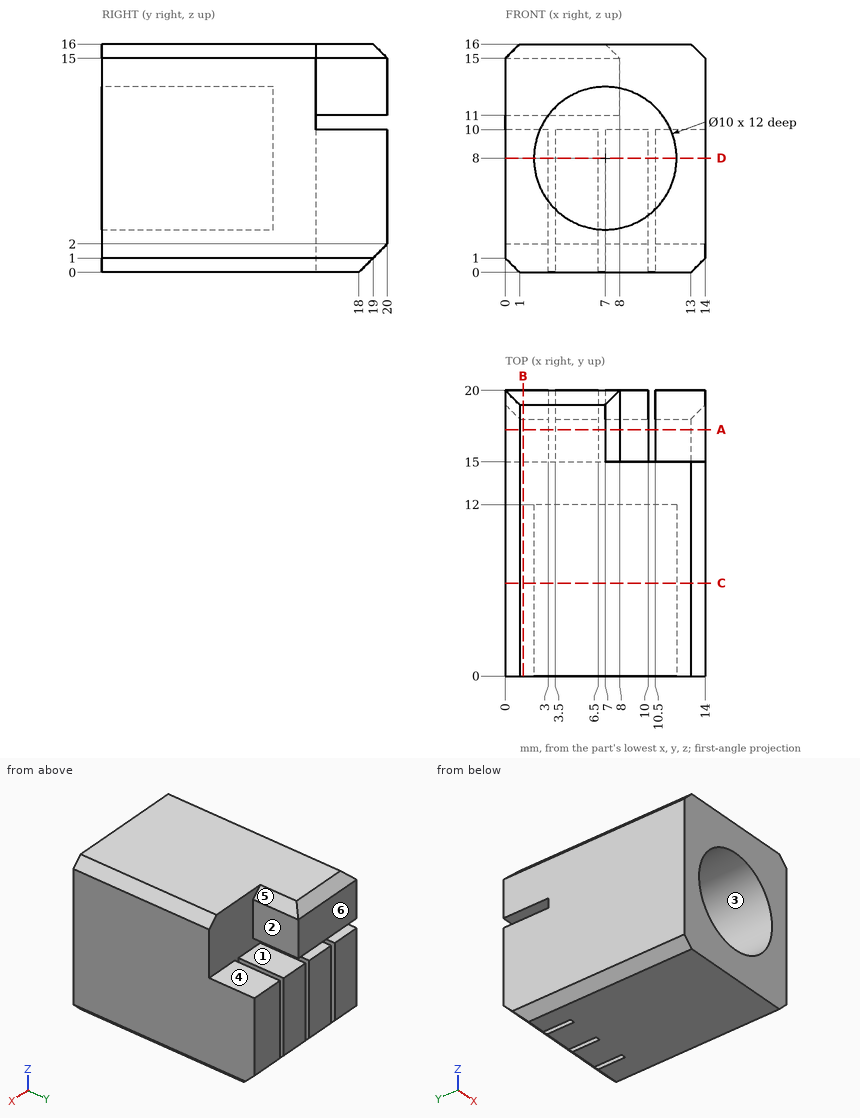
Job drawing, mm, ordinate dimensions from the low corner. One solid piece. A direction names the side the tool comes from. Round coordinates to 2 decimals unless told otherwise and drop trailing zeros. Loops run counter-clockwise (first coordinate to the right, second up) from the corner with the lowest first, then second, coordinate; pieces in that order, holes last. Notation, with made-up numbers: M -11.75,85.5 L 13.25,85.5 A14 cw 13.25,96.5 Z; hole C 15,-12.75 d2. An arc over 180 degrees is marked long. One line per question, with ' | ' between items. Start each with the question number.
Item 1: Two-plate mould, pull along X, no slides. Class the marked faces 1, 2 and 3: pulls with the +X half, pulls with the -X half, needs draft (parallel to the pull), parting line crosses it, or undercut.
Item 2: Pin check, flat tips, straight feed: pin 1 Ø1.8 at (x, y) = (12.5, 16.5) entering from +Z; pin 2 Ø5 at (x, y) = (4.5, 9.5) entering from -Z; pin 3 Ø1.5 at (x, z) = (11.5, 12) entering from +Y; pin 4 Ø3 at (y, z) = (18, 13.5) entering from +X. Stop position of each tip, or through.
Item 3: Which spindle directions (+Z, -Z, +X, -X, +Y, -Y) get a long thin tool onto all of the face, cutting with end or side? Do the marked faces 4, 5 and 6. Say none if no direction does.
Item 4: Cut at B-B, the plane x = 1.25. Write the cut outline in (y, z).
Item 5: Cut at A-A, the plane y = 17.25. Write the cut outline in (x, z), plus the area to 3 significant figures.
Item 6: Wall check: line 1 (X direction, y = 5.5, z = 8.25); line 2 (Z direction, x = 3, y = 2.5); line 3 (X direction, y = 3.5, z = 10.75). Give the ranges that are in metal, low to high.
Item 7: Cut at C-C, the plane y = 6.5. Write the cut outline in (x, z).
Item 8: Cut at D-D, the plane z = 8. Write the cut outline in (x, y).
Responses:
1) face 1: needs draft | face 2: pulls with the +X half | face 3: undercut
2) pin 1: stops at z = 10 | pin 2: stops at z = 0 | pin 3: stops at y = 15 | pin 4: stops at x = 8
3) face 4: +Z, +X, -X, +Y | face 5: +Z, +X, +Y | face 6: +Z, -Z, +X, -X, +Y
4) outline: M 0,0 L 18,0 L 20,2 L 20,10 L 15,10 L 15,11 L 20,11 L 20,15 L 19,16 L 0,16 Z
5) outline: M 0,1 L 1,0 L 3,0 L 3,10 L 0,10 Z; M 0,11 L 8,11 L 8,15 L 7,16 L 1,16 L 0,15 Z; M 3.5,0 L 6.5,0 L 6.5,10 L 3.5,10 Z; M 7,0 L 10,0 L 10,10 L 7,10 Z; M 10.5,0 L 13,0 L 14,1 L 14,10 L 10.5,10 Z | area: 163 mm²
6) line 1: x = 0 to 2.01, 11.99 to 14 | line 2: z = 0 to 5, 11 to 16 | line 3: x = 0 to 2.82, 11.18 to 14
7) outline: M 0,1 L 1,0 L 13,0 L 14,1 L 14,15 L 13,16 L 1,16 L 0,15 Z; hole C 7,8 d10
8) outline: M 0,0 L 2,0 L 2,12 L 12,12 L 12,0 L 14,0 L 14,20 L 10.5,20 L 10.5,15 L 10,15 L 10,20 L 7,20 L 7,15 L 6.5,15 L 6.5,20 L 3.5,20 L 3.5,15 L 3,15 L 3,20 L 0,20 Z
